Model file for the job. Use its own axes, mm. Round coordinates to 2 decimals unless told otherwise and drop trailing zeros. Write each loop counter-clockwise with the first axis right and the second up, starting at its lowest first coordinate (ties: lowest second). Pieces come first, ordered by that corner, then holes.
```python
from build123d import *

# Parameters (mm, degrees)
SKETCH_1_W          = 7
SKETCH_1_H          = 24
EXTRUDE_1_DEPTH     = 8
SKETCH_2_R          = 6
CUT_EXTRUDE_1_DEPTH = 7
SKETCH_3_R          = 1.6
CUT_EXTRUDE_2_DEPTH = 27.248809497


with BuildPart() as part:
    # 草图1 → 凸台-拉伸1 (new body)
    with BuildSketch(Plane(origin=(0, 0, 0), x_dir=(1, 0, 0), z_dir=(0, 1, 0))):
        with Locations((3.5, -12)):
            Rectangle(SKETCH_1_W, SKETCH_1_H)
    extrude(amount=EXTRUDE_1_DEPTH)

    # 草图2 → 切除-拉伸1 (cut)
    with BuildSketch(Plane.ZY):
        with Locations((12, 0)):
            Circle(SKETCH_2_R)
    extrude(amount=-CUT_EXTRUDE_1_DEPTH, mode=Mode.SUBTRACT)

    # 草图3 → 切除-拉伸2 (cut, through all)
    with BuildSketch(Plane.XZ):
        with Locations(Location((3.5, 21, 0), (0, 0, 270))):
            Circle(SKETCH_3_R)
        with Locations(Location((3.5, 3, 0), (0, 0, 270))):
            Circle(SKETCH_3_R)
    extrude(amount=-CUT_EXTRUDE_2_DEPTH, mode=Mode.SUBTRACT)


solid = part.part
```
1) Cut at D-D on y = 7. List the corners of the cut face in (x, z).
2) Cut at C-C on x = 3.75. List the corners of the cut face in (y, z).
3) Pull direction Z, two halves, no side cores. Call faces 1 (the face through (2, 0, 20)), 2 (the face through (3, 4, 24)), 3 (the face through (3, 6, 12)): released by +Z, released by -Z, zero draft, split by the parting line, or undercut.
4) Cut at A-A on z = 21. List the corners of the cut face in (x, y), and give its area (3 significant figures).
5) Flat gauge pin, fed straight in: pin 1 Ø2 at (x, y) = (3.5, 3.5) entering from -Z. Where does the tip first touch, or does it go through?
6) Cut at B-B on y = 2.5. List the corners of the cut face in (x, z), and give its area (3 significant figures).
7) Wall check: probe 1 along X at (y, z) = (3, 3); probe 2 along Z at (x, y) = (3, 7.25); probe 3 along Z at (x, y) = (1.75, 2.75). Give the ranges that are in metal, low to high.
Result sheet:
1. outline: (0, 0) - (7, 0) - (7, 24) - (0, 24) - close; hole circle Ø3.2 at (3.5, 3); hole circle Ø3.2 at (3.5, 21)
2. outline: (0, 0) - (8, 0) - (8, 1.42) - (0, 1.42) - close; (0, 4.58) - (8, 4.58) - (8, 19.42) - (0, 19.42) - (0, 18) arc R6 cw to (0, 6) - close; (0, 22.58) - (8, 22.58) - (8, 24) - (0, 24) - close
3. face 1: zero draft
3. face 2: released by +Z
3. face 3: undercut
4. outline: (0, 0) - (1.9, 0) - (1.9, 8) - (0, 8) - close; (5.1, 0) - (7, 0) - (7, 8) - (5.1, 8) - close
4. area: 30.4 mm2
5. pin 1: stops at z = 0
6. outline: (0, 0) - (7, 0) - (7, 6.55) - (0, 6.55) - close; (0, 17.45) - (7, 17.45) - (7, 24) - (0, 24) - close; hole circle Ø3.2 at (3.5, 3); hole circle Ø3.2 at (3.5, 21)
6. area: 75.6 mm2
7. probe 1: x = 0 to 1.9, 5.1 to 7
7. probe 2: z = 0 to 1.48, 4.52 to 19.48, 22.52 to 24
7. probe 3: z = 0 to 6.67, 17.33 to 24
